The figure shows three views and two pictorial views of one solid part (mm, origin at its lowest corner). Answer the questions. A direction names the side the tool comes from. Coordinates: 2 decimals unless noted, no trailing zeros. Write each loop counter-clockwise with the first axis right and the second up, starting at its lowest first coordinate (ties: lowest second). Pieces come first, ordered by that corner, then holes. Notation, with made-up numbers: M -7,-4.5 L 24,-4.5 A30 cw 24,31.5 Z; hole C 27,82.5 d7. An arc over 180 degrees is marked long. Answer as CSV lines item,"result".
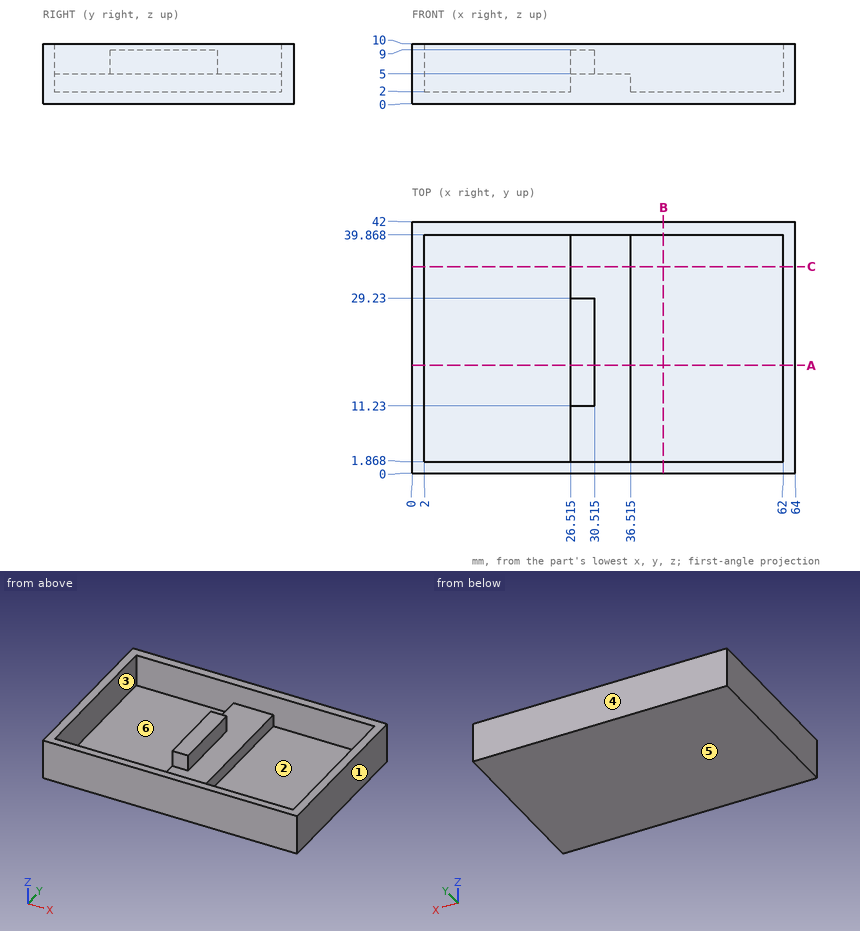
Q1. Find section B-B (x = 42). Give the vertices of the cut face in (y, z).
Output:
outline,"M 0,0 L 42,0 L 42,10 L 39.87,10 L 39.87,2 L 1.87,2 L 1.87,10 L 0,10 Z"
Q2. Flat-ended cylindrical pins translate along their axes: pin 1 Ø10 at (x, y) = (42, 31.5) entering from +Z; pin 2 Ø5 at (x, y) = (29.5, 30) entering from +Z; pin 3 Ø1.5 at (x, y) = (13.5, 12.5) entering from -Z. Find the tip coordinate at first contact, or state that the pin passes through.
Output:
pin 1,"z = 2"
pin 2,"z = 9"
pin 3,"z = 0"
Q3. For the marked faces 5 and 6, determine the directions among +Z, -Z, +X, -X, +Y, -Y from which every point of the face is accessible in a straight line to the end or side of a thin tool.
Output:
face 5,"-Z, +X, -X, +Y, -Y"
face 6,"+Z"
Q4. Straight lines are drawn through the part: line 1 (X direction, y = 26, z = 2.25) (1 decimal); line 2 (X direction, y = 25.5, z = 8.5) (1 decimal); line 3 (X direction, y = 32.5, z = 9.5). For each, find the intervals that lie inside material, in ascending order.
Output:
line 1,"0 to 2, 26.5 to 36.5, 62 to 64"
line 2,"0 to 2, 26.5 to 30.5, 62 to 64"
line 3,"0 to 2, 62 to 64"
Q5. Find section C-C (y = 34.5). Give the vertices of the cut face in (x, z) (1 decimal).
Output:
outline,"M 0,0 L 64,0 L 64,10 L 62,10 L 62,2 L 36.5,2 L 36.5,5 L 26.5,5 L 26.5,2 L 2,2 L 2,10 L 0,10 Z"
Q6. The mould has two halves that part along Y. Classify the marked faces 1, 2, 3 and 4: pulls with the +Y half, pulls with the -Y half, needs draft (parallel to the pull), parting line crosses it, or undercut.
Output:
face 1,"needs draft"
face 2,"undercut"
face 3,"undercut"
face 4,"pulls with the +Y half"
Q7. Find section A-A (y = 18). Give the vertices of the cut face in (x, z) (1 decimal), and give its area (3 significant figures).
Output:
outline,"M 0,0 L 64,0 L 64,10 L 62,10 L 62,2 L 36.5,2 L 36.5,5 L 30.5,5 L 30.5,9 L 26.5,9 L 26.5,2 L 2,2 L 2,10 L 0,10 Z"
area,"206 mm2"
